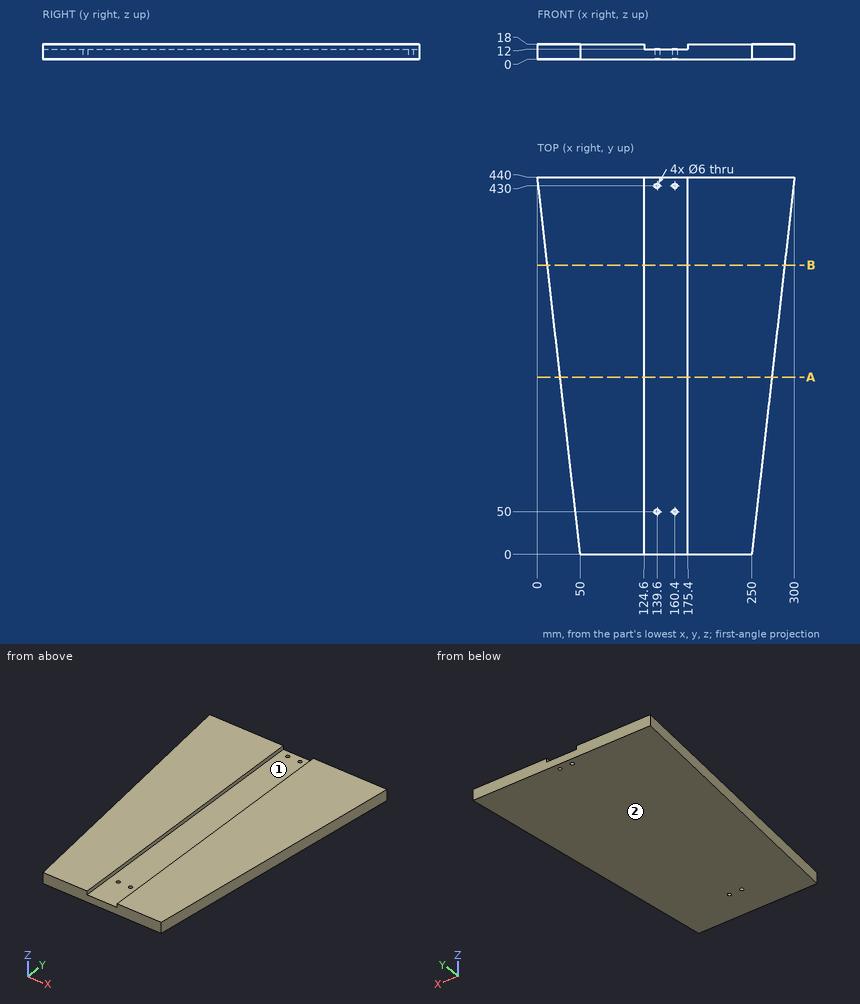
Here's the drawing with two shaded views (mm, measured from the low corner). I have some questions. Give positions to 0.01 mm unless a question says otherwise; leave off trailing zeros. Loops run counter-clockwise (first coordinate to the right, second up) from the corner with the lowest first, then second, coordinate; pieces in that order, holes last. Notation, with made-up numbers: M 8.25,-24 L 51.25,-24 A36 ccw 51.25,11 Z; hole C 67,25.25 d8. An arc over 180 degrees is marked long. One line per item, written item: value. Start each with the question number.
1) If I drill on line 1 (Y direction, x = 139.6, z = 6.5); line 2 (Z direction, x = 129, y = 348.5); line 3 (X direction, y = 188.5, z = 6.5), over which ranges is the centre line in solid material (lowest first)? Write a range as [from, to].
2) I'm going to push flat-ended pins straight in: pin 1 (8 mm diameter, centred on y = 96, z = 5, fed in from -X); pin 2 (3 mm diameter, centred on y = 154.5, z = 13.5, fed in from +X); pin 3 (8 mm diameter, centred on x = 139.6, y = 50, fed in from +Z). Where does each tip first touch, or does it pass through?
3) If we section it at A-A, the plane y = 207: Write out the boundary of the cut face in (x, z).
4) Thinking about a two-plate mould opening in X: for the marked faces 1 and 2, which applies, +X half, -X half, draft (parallel to the pull), parting line (faces both ways), or undercut?
5) If we section it at B-B, the plane y = 337.5: Write out the boundary of the cut face in (x, z).
Completed:
1. line 1: y = [0, 47], [53, 427], [433, 440]
1. line 2: z = [0, 12]
1. line 3: x = [28.58, 271.42]
2. pin 1: stops at x = 38.64
2. pin 2: stops at x = 267.73
2. pin 3: stops at z = 12
3. outline: M 26.48,0 L 273.52,0 L 273.52,18 L 175.4,18 L 175.4,12 L 124.6,12 L 124.6,18 L 26.48,18 Z
4. face 1: undercut
4. face 2: draft
5. outline: M 11.65,0 L 288.35,0 L 288.35,18 L 175.4,18 L 175.4,12 L 124.6,12 L 124.6,18 L 11.65,18 Z
